from build123d import *

# Parameters (mm, degrees)
BOSS_EXTRUDE1_DEPTH = 3
CUT_EXTRUDE1_DEPTH  = 56.554387766
SKETCH3_R           = 2
CUT_EXTRUDE2_DEPTH  = 56.554387766


with BuildPart() as part:
    # Sketch1 → Boss-Extrude1 (new body)
    with BuildSketch(Plane(origin=(0, 0, 0), x_dir=(1, 0, 0), z_dir=(0, 1, 0))):
        Polygon((-50.8, -5), (-50.8, -12.7), (50.8, -12.7), (50.8, -5), (54, -5), (54, 5), (50.8, 5), (50.8, 12.7), (-50.8, 12.7), (-50.8, 5), (-54, 5), (-54, -5), align=None)
    extrude(amount=BOSS_EXTRUDE1_DEPTH)

    # Sketch2 → Cut-Extrude1 (cut, through all)
    with BuildSketch(Plane(origin=(0, 3, 0), x_dir=(1, 0, 0), z_dir=(0, 1, 0))):
        with BuildLine():
            ThreePointArc((2.927112115, -7.445267938), (4.175733356, -6.823727057), (5.297427434, -5.994769602))
            ThreePointArc((5.297427434, -5.994769602), (6.708952064, -6.081937373), (6.621784293, -7.493462002))
            ThreePointArc((6.621784293, -7.493462002), (5.219666694, -8.529658821), (3.658890144, -9.306584922))
            ThreePointArc((3.658890144, -9.306584922), (2.362342638, -8.741815444), (2.927112115, -7.445267938))
        make_face()
        with BuildLine():
            ThreePointArc((-3.658890144, 9.306584922), (-5.219666694, 8.529658821), (-6.621784293, 7.493462002))
            ThreePointArc((-6.621784293, 7.493462002), (-6.708952064, 6.081937373), (-5.297427434, 5.994769602))
            ThreePointArc((-5.297427434, 5.994769602), (-4.175733356, 6.823727057), (-2.927112115, 7.445267938))
            ThreePointArc((-2.927112115, 7.445267938), (-2.362342638, 8.741815444), (-3.658890144, 9.306584922))
        make_face()
    extrude(amount=-CUT_EXTRUDE1_DEPTH, mode=Mode.SUBTRACT)

    # Sketch3 → Cut-Extrude2 (cut, through all)
    with BuildSketch(Plane(origin=(0, 3, 0), x_dir=(1, 0, 0), z_dir=(0, 1, 0))):
        with Locations(Location((29, 0, 0), (0, 0, 270))):
            Circle(SKETCH3_R)
        with Locations(Location((-29, 0, 0), (0, 0, 270))):
            Circle(SKETCH3_R)
    extrude(amount=-CUT_EXTRUDE2_DEPTH, mode=Mode.SUBTRACT)


solid = part.part
CAD build for the part. Positions are in the model's coordinates, mm. A direction names the side the tool comes from. Round coordinates to 2 decimals unless told otherwise and drop trailing zeros. Write each loop counter-clockwise with the first axis right and the second up, starting at its lowest first coordinate (ties: lowest second). Pieces come first, ordered by that corner, then holes. Notation, with made-up numbers: M 79,-17.5 L 119,-17.5 A24 cw 119,-6.5 Z; hole C 50,27.5 d8. An arc over 180 degrees is marked long. Put each result on its own line as item: value. Start each with the question number.
1) Pin check, flat tips, straight feed: pin 1 Ø0.9 at (x, y) = (-52, 1) entering from +Z; pin 2 Ø1.5 at (x, y) = (52, 1.5) entering from -Z; pin 3 Ø0.9 at (y, z) = (1.5, 9.5) entering from +X. Stop position of each tip, or through.
2) 3-axis set-ups, long thin cutter, end or side, ignore diameter. For faces 1 (the flat face through (-50.8, 1, 9)), 2 (the cylindrical face through (-5.2, 1.52, -8.54)), 3 (the flat face through (52, 1, 5)): which of +Z, -Z, +X, -X, +Y, -Y reach the whole face in a straight line?
3) Drill centre lines: probe 1 along X at (y, z) = (1.3, 0); probe 2 along X at (y, z) = (1.9, 10.5); probe 3 along X at (y, z) = (2.4, -6.5). Where is each one in solid material? Low to high. Write a range as [from, to].
4) Saw through at B-B, the plane z = 0. Write the cut outline in (x, y).
5) Pull direction X, two halves, no side cores. Call faces 4 (the cylindrical face through (-31, 2, 0)), 5 (the flat face through (50.8, 1, 9)), 6 (the flat face through (-50.8, 1, -9)): pulls with the +X half, pulls with the -X half, needs draft (parallel to the pull), parting line crosses it, or undercut.
6) Saw through at C-C, the plane y = 0.65. Write the cut outline in (x, z), and give its area (3 significant figures).
7) Saw through at A-A, the plane x = -29. Write the cut outline in (y, z).
Resolved:
1. pin 1: z = 5
1. pin 2: z = -5
1. pin 3: x = 50.8
2. face 1: +Z, -X, +Y, -Y
2. face 2: +Y, -Y
2. face 3: +Z, +X, +Y, -Y
3. probe 1: [-54, -31], [-27, 27], [31, 54]
3. probe 2: [-50.8, 50.8]
3. probe 3: [-50.8, -6.93], [-4.66, 50.8]
4. outline: M -54,0 L -31,0 L -31,3 L -54,3 Z; M -27,0 L 27,0 L 27,3 L -27,3 Z; M 31,0 L 54,0 L 54,3 L 31,3 Z
5. face 4: undercut
5. face 5: pulls with the +X half
5. face 6: pulls with the -X half
6. outline: M -54,-5 L -50.8,-5 L -50.8,-12.7 L 50.8,-12.7 L 50.8,-5 L 54,-5 L 54,5 L 50.8,5 L 50.8,12.7 L -50.8,12.7 L -50.8,5 L -54,5 Z; hole C -29,0 d4; hole M -6.62,-7.49 A10 ccw -3.66,-9.31 A1 ccw -2.93,-7.45 A8 cw -5.3,-5.99 A1 ccw Z; hole M 2.93,7.45 A8 cw 5.3,5.99 A1 ccw 6.62,7.49 A10 ccw 3.66,9.31 A1 ccw Z; hole C 29,0 d4
6. area: 2,600 mm²
7. outline: M 0,-12.7 L 3,-12.7 L 3,-2 L 0,-2 Z; M 0,2 L 3,2 L 3,12.7 L 0,12.7 Z
